Can you work these out from the drawing? Everything is in mm from the part's minimum corner. A direction names the side the tool comes from. Round coordinates to 2 decimals unless told otherwise and drop trailing zeros. Write each loop counter-clockwise with the first axis right and the second up, starting at its lowest first coordinate (ties: lowest second). Pieces come first, ordered by that corner, then holes. Notation, with made-up numbers: (3, -18) -> (36, -18) arc R15 ccw to (36, -4) -> close; hole circle Ø2 at (-22.75, 45). An arc over 180 degrees is marked (long way). Write item = value, one per line. Start each with the question number.
1) For the marked faces 1 and 2, which set-ups out of +Z, -Z, +X, -X, +Y, -Y let a thin tool reach every point of the face, with its end or its side?
2) Imagine slicing it at A-A, the plane z = 52.5. Please give me the cut outline in (x, y) (3 decimals).
3) Imagine slicing it at B-B, the plane y = 3.81. Please give me the cut outline in (x, z), then the cut area to 3 significant figures.
4) If I drill on line 1 (Z direction, x = 10.5, y = 26.5); line 2 (X direction, y = 15, z = 14); line 3 (Z direction, x = 26.5, y = 4.5), over which ranges is the centre line in solid material (lowest first)?
5) Imagine slicing it at C-C, the plane x = 11. Please give me the cut outline in (y, z).
6) Imagine slicing it at D-D, the plane y = 13. Please give me the cut outline in (x, z), then the cut area to 3 significant figures.
7) I'm going to push flat-ended pins straight in: pin 1 (1.5 mm diameter, centred on x = 21, y = 24, fed in from +Z); pin 2 (1.5 mm diameter, centred on x = 18.5, y = 18, fed in from +Z). Where does each tip first touch, or does it pass through?
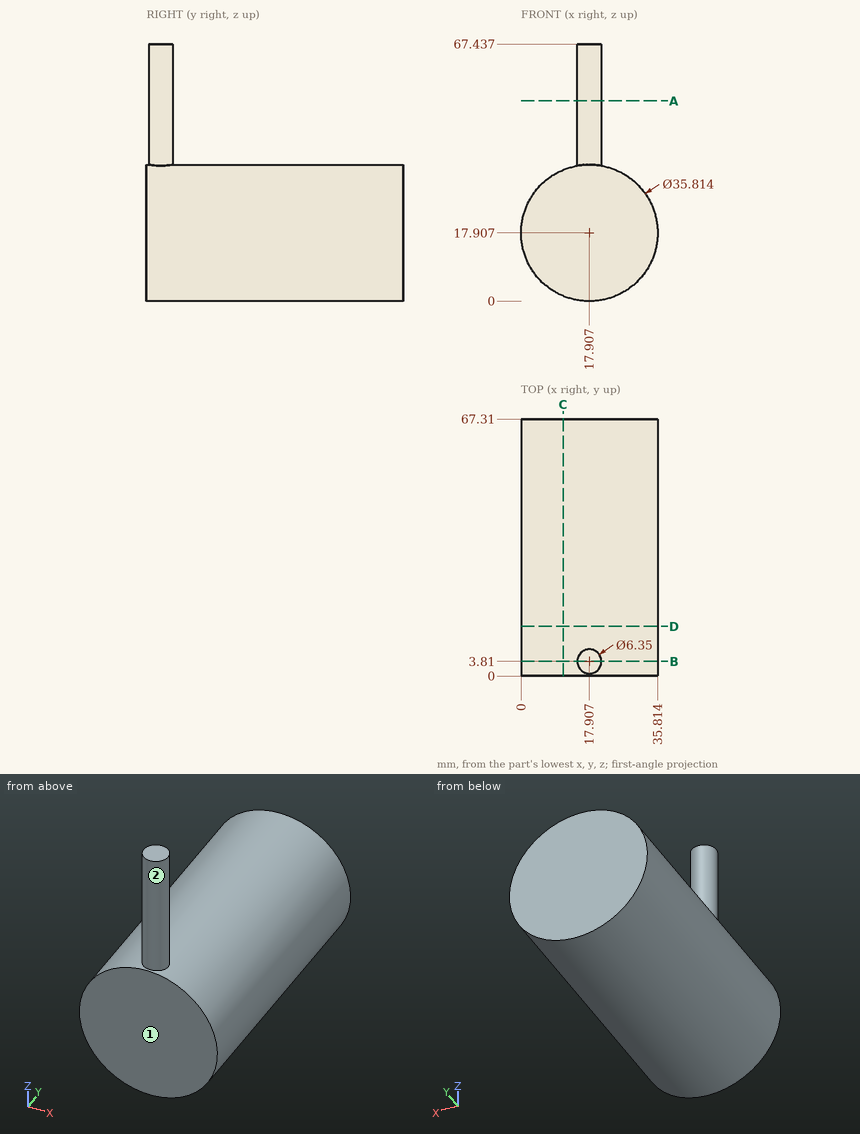
Reported:
q1.face_1 = +Z, -Z, +X, -X, -Y
q1.face_2 = +Z
q2.outline = circle Ø6.35 at (17.907, 3.81)
q3.outline = (14.73, 35.53) arc R17.91 ccw (long way) to (21.08, 35.53) -> (21.08, 67.44) -> (14.73, 67.44) -> close
q3.area = 1,210 mm²
q4.line_1 = 1.6 to 34.21
q4.line_2 = 0.43 to 35.38
q4.line_3 = 2.2 to 33.62
q5.outline = (0, 1.39) -> (67.31, 1.39) -> (67.31, 34.43) -> (0, 34.43) -> close
q6.outline = circle Ø35.81 at (17.91, 17.91)
q6.area = 1,010 mm²
q7.pin_1 = 35.66
q7.pin_2 = 35.81
